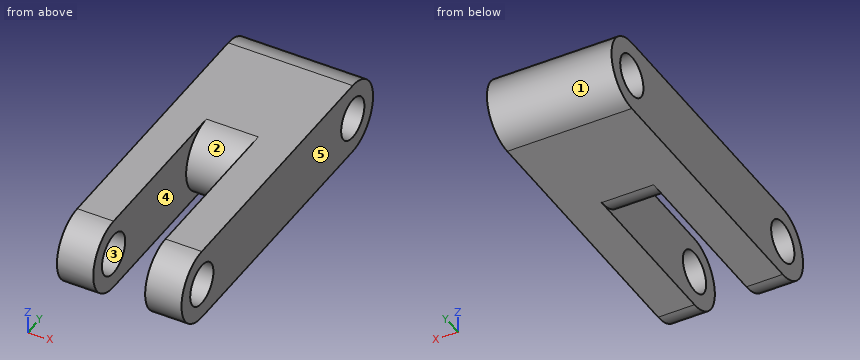
```python
from build123d import *

# Parameters (mm, degrees)
EXTRUDE_1_DEPTH     = 12
SKETCH_2_R          = 2
CUT_EXTRUDE_2_DEPTH = 15
CUT_EXTRUDE_3_DEPTH = 5


with BuildPart() as part:
    # Эскиз1 → Бобышка-Вытянуть1 (new body)
    with BuildSketch(Plane(origin=(0, 0, 0), x_dir=(0, 0, -1), z_dir=(1, 0, 0))):
        with BuildLine():
            Line((0, 0), (0, 26))
            ThreePointArc((0, 26), (3.5, 29.5), (7, 26))
            Line((7, 26), (7, 0))
            ThreePointArc((7, 0), (3.5, -3.5), (0, 0))
        make_face()
    extrude(amount=EXTRUDE_1_DEPTH)

    # Эскиз2 → Вырез-Вытянуть2 (cut)
    with BuildSketch(Plane(origin=(12, 0, 0), x_dir=(0, 0, -1), z_dir=(1, 0, 0))):
        with Locations((3.5, 0)):
            Circle(SKETCH_2_R)
        with Locations((3.5, 26)):
            Circle(SKETCH_2_R)
    extrude(amount=-CUT_EXTRUDE_2_DEPTH, mode=Mode.SUBTRACT)

    # Эскиз3 → Вырез-Вытянуть3 (cut)
    with BuildSketch(Plane(origin=(3.5, 0, 0), x_dir=(0, 0, -1), z_dir=(1, 0, 0))):
        with BuildLine():
            Line((0, 16), (-8.33598626, 16))
            Line((-8.33598626, 16), (-8.33598626, -12.274921498))
            Line((-8.33598626, -12.274921498), (16.66401374, -12.274921498))
            Line((16.66401374, -12.274921498), (16.66401374, 16))
            Line((16.66401374, 16), (7, 16))
            ThreePointArc((7, 16), (3.5, 12.5), (0, 16))
        make_face()
    extrude(amount=CUT_EXTRUDE_3_DEPTH, mode=Mode.SUBTRACT)


solid = part.part
```
Here's how the part is built. I have some questions about the finished solid (model axes, mm). Face numbers are marked on the shaded views. A direction names the side the tool comes from. Give positions to 0.01 mm unless a question says otherwise; leave off trailing zeros. Order: outer loops, then holes, each group sorted by start corner. A loop starts at its lowest first (then second) coordinate and runs counter-clockwise, first axis right, second up. Notation, with made-up numbers: M 79,52.5 L 105,52.5 A26 ccw 105,76.5 Z; hole C 40,4.5 d2. An arc over 180 degrees is marked long. Use a Markdown table: item, result. Add a question column.
1. I need wall thicknesses on probe 1 along Y at (x, z) = (1.7, -3.5); probe 2 along Y at (x, z) = (6.25, -3.5); probe 3 along X at (y, z) = (11, -1.5). Which ranges of each line are inside material? Lowest first, please. Write a range as from..to.
2. On a 3-axis mill with a long thin cutter (end or side, diameter ignored), from which of +Z, -Z, +X, -X, +Y, -Y can I reach the whole of each face in a straight line? I mean the marked faces 1 and 2. Say none if no direction works.
3. Suppose I cut it at C-C (x = 5.5). List the corners of the cut face in (y, z) for me.
4. Suppose I cut it at B-B (y = 5.5). List the corners of the cut face in (x, z) for me, and give its area (3 significant figures).
5. Suppose I cut it at D-D (z = -0.75). List the corners of the cut face in (x, y) for me, and give its area (3 significant figures).
6. For pin 1 Ø4 at (x, z) = (5, -3) entering from -Y, with a flat end and sliding along its axis, tell me the tip position at first contact or that it passes through.
7. If we mould it in two halves opening along X, with no side actions, what happens to the marked faces 3, 4 and 5? For each: +X half, -X half, draft (parallel to the pull), parting line (faces both ways), or undercut.
8. Suppose I cut it at A-A (z = -3.5). List the corners of the cut face in (x, y) for me, and give its area (3 significant figures).
Results list:
| question | item | result |
|---|---|---|
| 1 | probe 1 | y = -3.5..-2, 2..24, 28..29.5 |
| 1 | probe 2 | y = 12.5..24, 28..29.5 |
| 1 | probe 3 | x = 0..3.5, 8.5..12 |
| 2 | face 1 | +X, -X, +Y |
| 2 | face 2 | -Y |
| 3 | outline | M 16,-7 L 26,-7 A3.5 ccw 26,0 L 16,0 A3.5 ccw Z; hole C 26,-3.5 d4 |
| 4 | outline | M 0,-7 L 3.5,-7 L 3.5,0 L 0,0 Z; M 8.5,-7 L 12,-7 L 12,0 L 8.5,0 Z |
| 4 | area | 49.0 mm² |
| 5 | outline | M 0,-2.17 L 3.5,-2.17 L 3.5,13.83 L 8.5,13.83 L 8.5,-2.17 L 12,-2.17 L 12,28.17 L 0,28.17 Z |
| 5 | area | 284 mm² |
| 6 | pin 1 | stops at y = -3.5 |
| 7 | face 3 | draft |
| 7 | face 4 | undercut |
| 7 | face 5 | +X half |
| 8 | outline | M 0,-3.5 L 3.5,-3.5 L 3.5,-2 L 0,-2 Z; M 0,2 L 3.5,2 L 3.5,12.5 L 8.5,12.5 L 8.5,2 L 12,2 L 12,24 L 0,24 Z; M 0,28 L 12,28 L 12,29.5 L 0,29.5 Z; M 8.5,-3.5 L 12,-3.5 L 12,-2 L 8.5,-2 Z |
| 8 | area | 240 mm² |
